Verification items for the finished model (mm, model axes). A direction names the side the tool comes from. Round coordinates to 2 decimals unless told otherwise and drop trailing zeros. Write each loop counter-clockwise with the first axis right and the second up, starting at its lowest first coordinate (ties: lowest second). Pieces come first, ordered by that corner, then holes. Notation, with made-up numbers: M 28,17 L 61,17 A14 ccw 61,41 Z; hole C 12,48.5 d10. An arc over 180 degrees is marked long. One line per question, with ' | ' between items.
Autodesk Inventor part; units mm, degrees
ref_plane "YZ Plane" through (0, 0, 0) normal (1, 0, 0) x (0, 1, 0)
ref_plane "XZ Plane" through (0, 0, 0) normal (0, 1, 0) x (-1, 0, 0)
ref_plane "XY Plane" through (0, 0, 0) normal (0, 0, 1) x (1, 0, 0)
sketch "Sketch1" plane through (0, 0, 0) normal (0, 1, 0) x (-1, 0, 0)
  line L0 (0, 7.3323) -> (6.35, 3.6662)
  line L1 (6.35, 3.6662) -> (6.35, -3.6662)
  line L2 (6.35, -3.6662) -> (0, -7.3323)
  line L3 (0, -7.3323) -> (-6.35, -3.6662)
  line L4 (-6.35, -3.6662) -> (-6.35, 3.6662)
  line L5 (-6.35, 3.6662) -> (0, 7.3323)
  point P0 (0, 0)
  point P1 (0, 0)
  dimension "d0" = 12.7
extrude "Extrusion1" add sketch "Sketch1" along normal blind 28.5242
sketch "Sketch2" plane through (0, 28.5242, 0) normal (0, 1, 0) x (1, 0, 0)
  circle A0 centre (0, 0) radius 2.0193
  dimension "d3" = 4.0386
extrude "Extrusion2" cut sketch "Sketch2" against normal blind 12.7
sketch "Sketch3" plane through (0, 0, 0) normal (0, -1, 0) x (1, 0, 0)
  circle A0 centre (0, 0) radius 2.0193
  dimension "d6" = 4.0386
extrude "Extrusion3" cut sketch "Sketch3" against normal blind 12.7
thread "Thread1"
thread "Thread2"
properties part number "DTraining2_001_E1Shaft"
1. Tool access check on faces 1 (the face through (2, 0, -2)), 2 (the face through (1.926, 22.263, -0.607)), 3 (the face through (0, 12.7, 0)). Record the directions out of +Z, -Z, +X, -X, +Y, -Y that give a thin tool (end or side, any length) a straight path to the whole face; none if there is none.
Results:
face 1: +Z, -Z, +X, -X, -Y | face 2: +Y | face 3: -Y
2. Section check A-A, the plane y = 25. Record the cut outline in (x, z).
Results:
outline: M -6.35,-3.67 L 0,-7.33 L 6.35,-3.67 L 6.35,3.67 L 0,7.33 L -6.35,3.67 Z; hole C 0,0 d4.04
3. Mould release check, pull along X, two halves, no side actions. Record for faces 4 (the face through (2, 28.524, -2)), 5 (the face through (-6.35, 14, 0)), 6 (the face through (0, 15.824, 0)): pulls with the +X half, pulls with the -X half, needs draft (parallel to the pull), parting line crosses it, or undercut.
Results:
face 4: needs draft | face 5: pulls with the -X half | face 6: undercut
4. Section check C-C, the plane x = 1.5. Record the cut outline in (y, z).
Results:
outline: M 0,-6.47 L 28.52,-6.47 L 28.52,-1.35 L 15.82,-1.35 L 15.82,1.35 L 28.52,1.35 L 28.52,6.47 L 0,6.47 L 0,1.35 L 12.7,1.35 L 12.7,-1.35 L 0,-1.35 Z
5. Thickness scan on line 1 (X direction, y = 25.75, z = 0); line 2 (Z direction, x = -0.75, y = 9); line 3 (Z direction, x = -1.5, y = 16). Record the ranges inside material, lowest first.
Results:
line 1: x = -6.35 to -2.02, 2.02 to 6.35 | line 2: z = -6.9 to -1.87, 1.87 to 6.9 | line 3: z = -6.47 to -1.35, 1.35 to 6.47
6. Section check D-D, the plane y = 14. Record the cut outline in (x, z).
Results:
outline: M -6.35,-3.67 L 0,-7.33 L 6.35,-3.67 L 6.35,3.67 L 0,7.33 L -6.35,3.67 Z
7. Section check B-B, the plane z = 0. Record the cut outline in (x, y), then the cut area to 3 significant figures.
Results:
outline: M -6.35,0 L -2.02,0 L -2.02,12.7 L 2.02,12.7 L 2.02,0 L 6.35,0 L 6.35,28.52 L 2.02,28.52 L 2.02,15.82 L -2.02,15.82 L -2.02,28.52 L -6.35,28.52 Z | area: 260 mm2
8. Go/stop test with flat-tipped pins: P1, Ø1.5, axis at x = 4, y = 17, coming from the +Z side; P2, Ø1.5, axis at y = 19.5, z = 5, coming from the -X side; P3, Ø4, axis at x = 4.5, y = 24.5, coming from the +Z side; P4, Ø4.5, axis at x = 0, z = 0, coming from the +Y side. Record where each tip stops, or that it passes through.
Results:
P1: stops at z = 5.46 | P2: stops at x = -5.34 | P3: stops at z = 5.89 | P4: stops at y = 28.52
